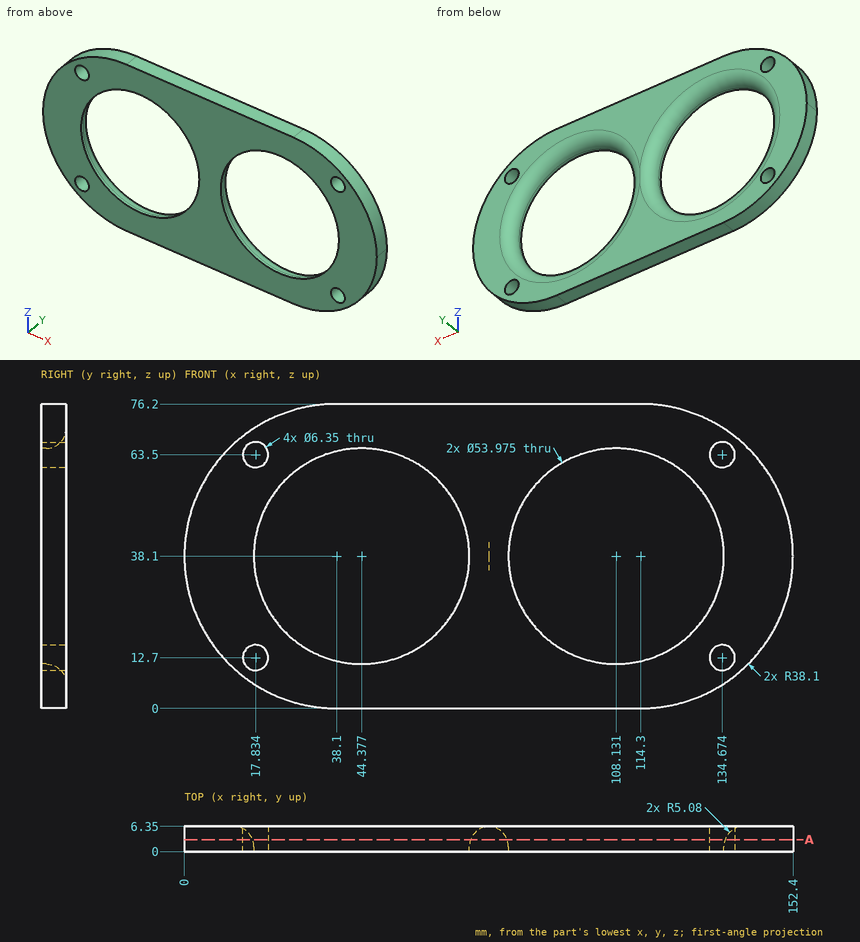
Input: dimensioned drawing with shaded views. Units: mm. Origin: part minimum x, y, z. Coordinates: 2 decimals unless noted, no trailing zeros.
1. Ray query, line 1 along X through (y, z) = (2.5, 66) (1 decimal); line 2 along X through (y, z) = (5.25, 45.5) (1 decimal); line 3 along Z through (x, y) = (42, 2.5). Return the intervals inside material, ascending.
Checked values:
line 1: x = 12.2 to 15.9, 19.8 to 132.7, 136.6 to 140.2
line 2: x = 0.7 to 16.4, 72.3 to 80.2, 136.1 to 151.7
line 3: z = 0 to 11.07, 65.13 to 76.2
2. Contact query for flat-ended pins moving along their axis: P1, Ø3, axis at x = 20, y = 2, coming from the -Z side; P2, Ø1, axis at x = 33, y = 4.5, coming from the -Z side; P3, Ø4, axis at x = 17.83, z = 63.5, coming from the -Y side (3 decimals). Output: stop coordinate, or through.
Checked values:
P1: stops at z = 3.81
P2: stops at z = 0.28
P3: passes through
3. Cut plane A-A, the plane y = 3. Count the separate pieces of the cut face and the enclosed holes in it, plus the area to 3 significant figures.
Checked values:
separate pieces: 1
enclosed holes: 6
area: 5,560 mm2
